The listing builds one solid part. Answer for the finished solid, in the listing's coordinates (mm). A direction names the side the tool comes from. Give positions to 0.01 mm unless a question says otherwise; leave off trailing zeros. Order: outer loops, then holes, each group sorted by start corner. A loop starts at its lowest first (then second) coordinate and runs counter-clockwise, first axis right, second up. Notation, with made-up numbers: (67, 66.25) - (101, 66.25) arc R30 ccw to (101, 101.25) - close; hole circle Ø5 at (-5, 79.25). An arc over 180 degrees is marked (long way). Use a Markdown table: item, result. Add a question column.
1) For faces 5 (the face through (45, 2, -18)), 6 (the face through (30, 12, 5)), 7 (the face through (17.5, 29, 2)), determine the directions among +Z, -Z, +X, -X, +Y, -Y from which every point of the face is accessible in a straight line to the end or side of a thin tool.
2) The mould has two halves that part along X. Classify faces 1 (the face through (41.844, 2.465, -17.628)), 2 (the face through (15, 2, -18)), 3 (the face through (50.253, 7.121, 2.465)), 4 (the face through (30, 5, -17)): released by +X, released by -X, zero draft, split by the parting line, or undercut.
3) Find section A-A, the plane y = 7. Determine the outline of the cut face in (x, z).
4) Find section D-D, the plane z = 1. Determine the outline of the cut face in (x, y).
5) Straight lines are drawn through the part: line 1 (X direction, y = 1.8, z = -16.15) (3 decimals); line 2 (Y direction, x = 53, z = 3.85); line 3 (X direction, y = 4, z = -27.5). For each, find the intervals that lie inside material, in ascending order.
6) Flat-ended cylindrical pins translate along their axes: pin 1 (2.5 mm diameter, centred on y = 2, z = -20.5, fed in from -X); pin 2 (9 mm diameter, centred on x = 7, y = 7, fed in from -Z); pin 3 (15 mm diameter, centred on x = 32, z = -17.5, fed in from +Y). Find the tip coordinate at first contact, or state that the pin passes through.
7) Find section C-C, the plane x = 40.5. Determine the outline of the cut face in (y, z).
8) Find section B-B, the plane z = -16.15. Determine the outline of the cut face in (x, y) (3 decimals).
from build123d import *

# Parameters (mm, degrees)
SKETCH1_R           = 2.75
BOSS_EXTRUDE1_DEPTH = 5
SKETCH2_W           = 30
SKETCH2_H           = 40
SKETCH2_R           = 2.75
BOSS_EXTRUDE2_DEPTH = 5


with BuildPart() as part:
    # Sketch1 → Boss-Extrude1 (new body)
    with BuildSketch(Plane.XY):
        with BuildLine():
            Line((0, 32.5), (0, 0))
            Line((0, 0), (60, 0))
            Line((60, 0), (60, 32.5))
            Line((60, 32.5), (42.5, 32.5))
            Line((42.5, 32.5), (42.5, 25))
            ThreePointArc((42.5, 25), (30, 12.5), (17.5, 25))
            Line((17.5, 25), (17.5, 32.5))
            Line((17.5, 32.5), (0, 32.5))
        make_face()
        with Locations((7, 7)):
            Circle(SKETCH1_R, mode=Mode.SUBTRACT)
        with Locations((53, 7)):
            Circle(SKETCH1_R, mode=Mode.SUBTRACT)
        with Locations((7, 25)):
            Circle(SKETCH1_R, mode=Mode.SUBTRACT)
        with Locations((53, 25)):
            Circle(SKETCH1_R, mode=Mode.SUBTRACT)
    extrude(amount=BOSS_EXTRUDE1_DEPTH)

    # Sketch2 → Boss-Extrude2 (add)
    with BuildSketch(Plane.XZ):
        with Locations((30, -15)):
            Rectangle(SKETCH2_W, SKETCH2_H)
        with Locations(Location((20.475, -16.15, 0), (0, 0, 270))):
            Circle(SKETCH2_R, mode=Mode.SUBTRACT)
        with Locations(Location((39.525, -16.15, 0), (0, 0, 270))):
            Circle(SKETCH2_R, mode=Mode.SUBTRACT)
        with Locations(Location((39.525, -28.85, 0), (0, 0, 270))):
            Circle(SKETCH2_R, mode=Mode.SUBTRACT)
        with Locations(Location((20.475, -28.85, 0), (0, 0, 270))):
            Circle(SKETCH2_R, mode=Mode.SUBTRACT)
    extrude(amount=-BOSS_EXTRUDE2_DEPTH)


solid = part.part
The answers:
| question | item | result |
|---|---|---|
| 1 | face 5 | -Z, +X, +Y, -Y |
| 1 | face 6 | +Z, +X, -X, +Y, -Y |
| 1 | face 7 | +Z, -Z, +Y |
| 2 | face 1 | undercut |
| 2 | face 2 | released by -X |
| 2 | face 3 | undercut |
| 2 | face 4 | zero draft |
| 3 | outline | (0, 0) - (4.25, 0) - (4.25, 5) - (0, 5) - close; (9.75, 0) - (50.25, 0) - (50.25, 5) - (9.75, 5) - close; (55.75, 0) - (60, 0) - (60, 5) - (55.75, 5) - close |
| 4 | outline | (0, 0) - (60, 0) - (60, 32.5) - (42.5, 32.5) - (42.5, 25) arc R12.5 cw to (17.5, 25) - (17.5, 32.5) - (0, 32.5) - close; hole circle Ø5.5 at (7, 7); hole circle Ø5.5 at (7, 25); hole circle Ø5.5 at (53, 7); hole circle Ø5.5 at (53, 25) |
| 5 | line 1 | 15 to 17.725, 23.225 to 36.775, 42.275 to 45 |
| 5 | line 2 | 0 to 4.25, 9.75 to 22.25, 27.75 to 32.5 |
| 5 | line 3 | 15 to 18.08, 22.87 to 37.13, 41.92 to 45 |
| 6 | pin 1 | x = 15 |
| 6 | pin 2 | z = 0 |
| 6 | pin 3 | y = 5 |
| 7 | outline | (0, -35) - (5, -35) - (5, -31.42) - (0, -31.42) - close; (0, -26.28) - (5, -26.28) - (5, -18.72) - (0, -18.72) - close; (0, -13.58) - (5, -13.58) - (5, 0) - (18.22, 0) - (18.22, 5) - (0, 5) - close |
| 8 | outline | (15, 0) - (17.725, 0) - (17.725, 5) - (15, 5) - close; (23.225, 0) - (36.775, 0) - (36.775, 5) - (23.225, 5) - close; (42.275, 0) - (45, 0) - (45, 5) - (42.275, 5) - close |
